from build123d import *

# Parameters (mm, degrees)
CYLINDER010_R     = 4.7
CYLINDER010_DEPTH = 10
CYLINDER009_R     = 3.5
CYLINDER009_DEPTH = 10
BOX004_W          = 15.9
BOX004_H          = 15.9
BOX004_DEPTH      = 2
CYLINDER008_R     = 5.3
CYLINDER008_DEPTH = 10
CHAMFER_SIZE      = 1
CHAMFER001_SIZE   = 1


with BuildPart() as lochschraubeoben:
    # Cylinder010 → Cylinder010 (new body)
    with BuildSketch(Plane.XY.offset(24)):
        Circle(CYLINDER010_R)
    extrude(amount=CYLINDER010_DEPTH)


with BuildPart() as zylinder:
    # Cylinder009 → Cylinder009 (new body)
    with BuildSketch(Plane.XY.offset(20)):
        Circle(CYLINDER009_R)
    extrude(amount=CYLINDER009_DEPTH)


with BuildPart() as obj1:
    # Box004 → Box004 (new body)
    with BuildSketch(Plane(origin=(-7.95, -7.95, 28), x_dir=(1, 0, 0), z_dir=(0, 0, 1))):
        with Locations((7.95, 7.95)):
            Rectangle(BOX004_W, BOX004_H)
    extrude(amount=BOX004_DEPTH)


with BuildPart() as bolt:
    # Cylinder008 → Cylinder008 (new body)
    with BuildSketch(Plane.XY.offset(20)):
        Circle(CYLINDER008_R)
    extrude(amount=CYLINDER008_DEPTH)

    # Fusion004: union obj1
    add(obj1.part)

    # Cut003: cut Zylinder
    add(zylinder.part, mode=Mode.SUBTRACT)

    # Cut004: cut LochSchraubeOben
    add(lochschraubeoben.part, mode=Mode.SUBTRACT)

    # Chamfer
    chamfer_edges = [bolt.edges().sort_by_distance(p)[0] for p in [
        (-3.5, 0, 24),
    ]]
    chamfer(chamfer_edges, length=CHAMFER_SIZE)

    # Chamfer001
    chamfer001_edges = [bolt.edges().sort_by_distance(p)[0] for p in [
        (-3.5, 0, 20),
    ]]
    chamfer(chamfer001_edges, length=CHAMFER001_SIZE)


solid = bolt.part
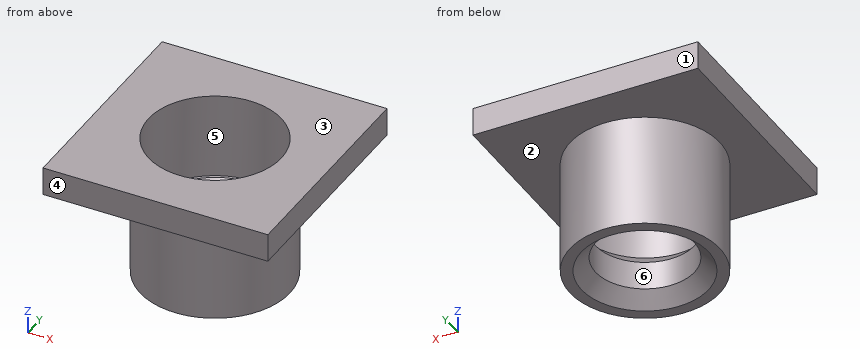
Input: part model. Units: mm. Frame: model coordinates. Face numbers are marked on the shaded views. A direction names the side the tool comes from. Coordinates: 2 decimals unless noted, no trailing zeros. Loops run counter-clockwise (first coordinate to the right, second up) from the corner with the lowest first, then second, coordinate; pieces in that order, holes last.
Q1. Cut plane D-D (z = 22.5). Output: boundary loops of the cut face in (x, y), then the cut area to 3 significant figures.
Q2. Material intervals for line 1 (X direction, y = 0, z = 22.6); line 2 (X direction, y = 0, z = 27.5); line 3 (Z direction, x = 3.25, y = -6), sorted ascending.
Q3. Contact query for flat-ended pins moving along their axis: pin 1 (1.5 mm diameter, centred on x = -4.5, z = 23, fed in from -Y); pin 2 (8 mm diameter, centred on x = 0, y = 0, fed in from -Z); pin 3 (2 mm diameter, centred on y = -0.5, z = 23, fed in from +X). Output: stop coordinate, or through.
Q4. Set-up query: the marked faces 1 and 2. Return all of +Z, -Z, +X, -X, +Y, -Y with unobstructed straight access to the full face (end or side cutting, diameter ignored); none if empty.
Q5. Cut plane C-C (z = 29). Output: boundary loops of the cut face in (x, y), then the cut area to 3 significant figures.
Q6. Draft query along Y for the marked faces 3, 4, 5 and 6. Return one class per face: +Y half, -Y half, draft (parallel to the pull), parting line (faces both ways), or undercut.
Q7. Cut plane A-A (x = 0). Output: boundary loops of the cut face in (y, z).
Working result:
1. outline: circle Ø10.6 at (0, 0); hole circle Ø7 at (0, 0)
1. area: 49.8 mm2
2. line 1: x = -5.3 to -3.5, 3.5 to 5.3
2. line 2: x = -5.3 to -4.7, 4.7 to 5.3
2. line 3: z = 28 to 30
3. pin 1: stops at y = -3.75
3. pin 2: stops at z = 20.5
3. pin 3: stops at x = 5.3
4. face 1: +Z, -Z, +X, -X, +Y
4. face 2: -Z
5. outline: (-7.95, -7.95) - (7.95, -7.95) - (7.95, 7.95) - (-7.95, 7.95) - close; hole circle Ø9.4 at (0, 0)
5. area: 183 mm2
6. face 3: draft
6. face 4: -Y half
6. face 5: undercut
6. face 6: undercut
7. outline: (-7.95, 28) - (-5.3, 28) - (-5.3, 20) - (-4.5, 20) - (-3.5, 21) - (-3.5, 23) - (-4.5, 24) - (-4.7, 24) - (-4.7, 30) - (-7.95, 30) - close; (3.5, 21) - (4.5, 20) - (5.3, 20) - (5.3, 28) - (7.95, 28) - (7.95, 30) - (4.7, 30) - (4.7, 24) - (4.5, 24) - (3.5, 23) - close
